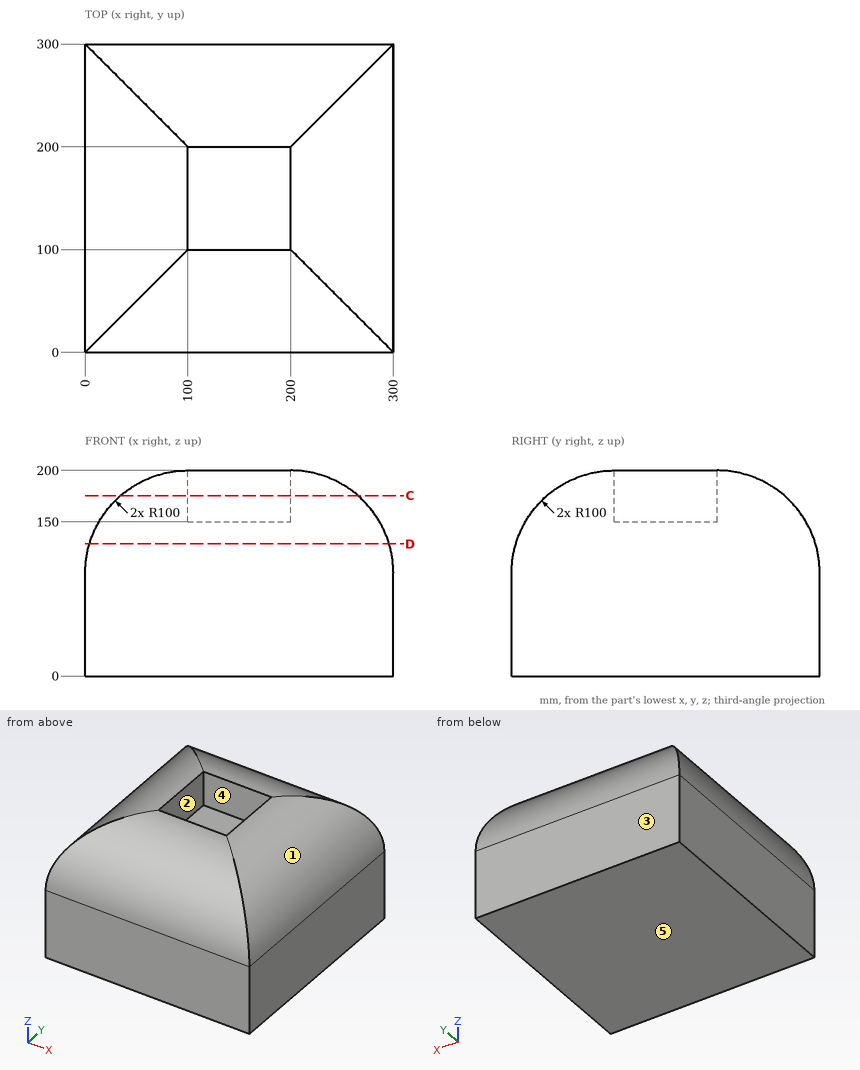
Can you work these out from the drawing? Everything is in mm from the part's minimum corner. A direction names the side the tool comes from. Round coordinates to 2 decimals unless told otherwise and drop trailing zeros. Loops run counter-clockwise (first coordinate to the right, second up) from the corner with the lowest first, then second, coordinate; pieces in that order, holes last.
1. Which directions (+Z, -Z, +X, -X, +Y, -Y) give clear straight access to the entire face, cutting with the end or side of a thin tool? Please do the marked faces 1 and 2.
Answer list:
face 1: +Z, +X, +Y, -Y
face 2: +Z
2. If I drill on line 1 along X through (y, z) = (162, 150.5); line 2 along Z through (x, y) = (132.5, 18); line 3 along Z through (x, y) = (280.5, 261), over which ranges is the centre line in solid material (lowest first)?
Answer list:
line 1: x = 13.69 to 100, 200 to 286.31
line 2: z = 0 to 157.24
line 3: z = 0 to 159.33
3. For P1, Ø2, axis at x = 125.5, y = 150, coming from the -Z side; P2, Ø3, axis at x = 194.5, z = 133.5, coming from the -Y side; P3, Ø3, axis at x = 95, y = 183.5, coming from the +Z side; P4, Ø1.5, axis at x = 132, z = 143, coming from the +Y side, each with a flat end and sliding along its axis, tell me the tip position at first contact or that it passes through.
Answer list:
P1: stops at z = 0
P2: stops at y = 5.26
P3: stops at z = 199.94
P4: stops at y = 290.64
4. We'd pull the mould along Y, two halves only. Please class the marked faces 3, 4 and 5: +Y half, -Y half, draft (parallel to the pull), parting line (faces both ways), or undercut.
Answer list:
face 3: +Y half
face 4: undercut
face 5: draft
5. If we section it at D-D on z = 128.5: Write out the boundary of the cut face in (x, y), plus the area to 3 significant figures.
Answer list:
outline: (4.15, 4.15) - (295.85, 4.15) - (295.85, 295.85) - (4.15, 295.85) - close
area: 85,100 mm2
6. If we section it at C-C on z = 175.5: Write out the boundary of the cut face in (x, y).
Answer list:
outline: (34.43, 34.43) - (265.57, 34.43) - (265.57, 265.57) - (34.43, 265.57) - close; hole (100, 100) - (200, 100) - (200, 200) - (100, 200) - close
